Verification items for this drawing (mm, ordinates from the low corner). Round coordinates to 2 decimals unless told otherwise and drop trailing zeros. Order: outer loops, then holes, each group sorted by start corner. A loop starts at its lowest first (then second) coordinate and runs counter-clockwise, first axis right, second up. Notation, with made-up numbers: (-34.5, 35.5) - (0.5, 35.5) arc R10 cw to (0.5, 53.5) - close; hole circle Ø2 at (-0.75, 51.25). An arc over 180 degrees is marked (long way). Answer as CSV lines item,"result". Start each with the question number.
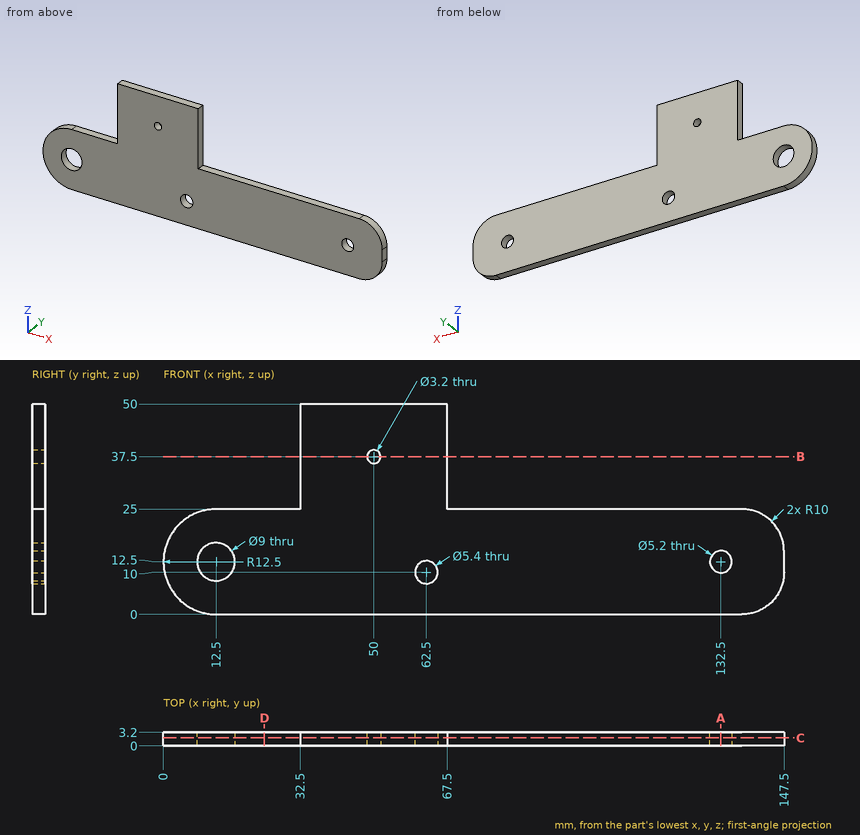
1. Section check D-D on x = 24. Record the boundary of the cut face in (y, z), plus the area to 3 significant figures.
2. Section check C-C on y = 1.9. Record the boundary of the cut face in (x, z), plus the area to 3 significant figures.
3. Section check B-B on z = 37.5. Record the boundary of the cut face in (x, y), plus the area to 3 significant figures.
4. Thickness scan on probe 1 along Z at (x, y) = (50, 1); probe 2 along Z at (x, y) = (62.5, 1.8); probe 3 along Z at (x, y) = (22, 2.05). Record the ranges inside material, lowest first.
5. Go/stop test with flat-tipped pins: pin 1 Ø1 at (y, z) = (2, 42) entering from -X; pin 2 Ø4 at (x, z) = (132.5, 12.5) entering from -Y; pin 3 Ø1 at (y, z) = (1, 33) entering from +X; pin 4 Ø1.6 at (x, y) = (25, 1.5) entering from +Z. Record where each tip stops, or that it passes through.
6. Section check A-A on x = 132.5. Record the boundary of the cut face in (y, z).
Numbers:
1,outline,"(0, 0) - (3.2, 0) - (3.2, 25) - (0, 25) - close"
1,area,"80.0 mm2"
2,outline,"(12.5, 0) - (137.5, 0) arc R10 ccw to (147.5, 10) - (147.5, 15) arc R10 ccw to (137.5, 25) - (67.5, 25) - (67.5, 50) - (32.5, 50) - (32.5, 25) - (12.5, 25) arc R12.5 ccw to start; hole circle Ø9 at (12.5, 12.5); hole circle Ø3.2 at (50, 37.5); hole circle Ø5.4 at (62.5, 10); hole circle Ø5.2 at (132.5, 12.5)"
2,area,"4,340 mm2"
3,outline,"(32.5, 0) - (48.4, 0) - (48.4, 3.2) - (32.5, 3.2) - close; (51.6, 0) - (67.5, 0) - (67.5, 3.2) - (51.6, 3.2) - close"
3,area,"102 mm2"
4,probe 1,"z = 0 to 35.9, 39.1 to 50"
4,probe 2,"z = 0 to 7.3, 12.7 to 50"
4,probe 3,"z = 0 to 25"
5,pin 1,"stops at x = 32.5"
5,pin 2,"passes through"
5,pin 3,"stops at x = 67.5"
5,pin 4,"stops at z = 25"
6,outline,"(0, 0) - (3.2, 0) - (3.2, 9.9) - (0, 9.9) - close; (0, 15.1) - (3.2, 15.1) - (3.2, 25) - (0, 25) - close"
